```python
from build123d import *

# Parameters (mm, degrees)
BOSS_EXTRUDE1_DEPTH = 38.1
CUT_EXTRUDE1_DEPTH  = 7.62
CUT_EXTRUDE4_DEPTH  = 39.624


with BuildPart() as part:
    # Sketch2 → Boss-Extrude1 (new body)
    with BuildSketch(Plane(origin=(0, 0, 0), x_dir=(1, 0, 0), z_dir=(0, 1, 0))):
        with BuildLine():
            Line((-13.549240888, -8.64489), (-13.549240888, -32.77489))
            Line((-13.549240888, -32.77489), (21.502759112, -26.594276672))
            Line((21.502759112, -26.594276672), (21.502759112, -40.52189))
            Line((21.502759112, -40.52189), (478.702759112, -40.52189))
            ThreePointArc((478.702759112, -40.52189), (498.514759112, -20.70989), (478.702759112, -0.89789))
            Line((478.702759112, -0.89789), (21.502759112, -0.89789))
            Line((21.502759112, -0.89789), (21.502759112, -14.825503328))
            Line((21.502759112, -14.825503328), (-13.549240888, -8.64489))
        make_face()
    extrude(amount=BOSS_EXTRUDE1_DEPTH)

    # Sketch3 → Cut-Extrude1 (cut)
    with BuildSketch(Plane(origin=(0, 38.1, 0), x_dir=(1, 0, 0), z_dir=(0, 1, 0))):
        Polygon((-13.549240888, -8.64489), (-13.549240888, -32.77489), (21.502759112, -26.594276672), (21.502759112, -14.825503328), align=None)
    extrude(amount=-CUT_EXTRUDE1_DEPTH, mode=Mode.SUBTRACT)

    # Sketch5 → Cut-Extrude4 (cut)
    with BuildSketch(Plane.XY.offset(40.52189)):
        Polygon((250.102759112, 38.1), (498.514759112, 15.775221318), (498.514759112, 38.1), align=None)
    extrude(amount=-CUT_EXTRUDE4_DEPTH, mode=Mode.SUBTRACT)


solid = part.part
```
Geometry check sheet. Reference: the model listing, model coordinates, mm. A direction names the side the tool comes from. Coordinates: 2 decimals unless noted, no trailing zeros. Order: outer loops, then holes, each group sorted by start corner. A loop starts at its lowest first (then second) coordinate and runs counter-clockwise, first axis right, second up. Notation, with made-up numbers: (2, 49.25) - (38, 49.25) arc R33 cw to (38, 78.25) - close; hole circle Ø1 at (21.25, 73.5). An arc over 180 degrees is marked (long way). Answer in a Markdown table with one row per item. Add a question column.
1. Draft check along X on faces 4 (the face through (372.57, 27.094, 20.987)), 5 (the face through (4.22, 15.03, 11.78)), 6 (the face through (239, 0, 20)). Enter one of: +X half, -X half, draft (parallel to the pull), parting line (faces both ways), or undercut.
2. Section check A-A (y = 10). Enter the section's corners in (x, z), plus the area to 3 significant figures.
3. Section check B-B (x = 362). Enter the section's corners in (y, z), plus the area to 3 significant figures.
4. Section check C-C (x = 418). Enter the section's corners in (y, z).
5. Material ranges on L1, parallel to Y at x = 335.5, z = 5; L2, parallel to X at y = 5.5, z = 20; L3, parallel to Y at x = 423.5, z = 37, recorded low to high. Write a range as [from, to].
6. Gauge pin test, flat end, axial feed: pin 1 Ø12 at (x, z) = (422, 35.5) entering from +Y. Record the tip position at first contact, or that the pin passes through.
7. Access from +Z, -Z, +X, -X, +Y, -Y to the whole of each face (thin tool, end or side, straight path). Record for faces 1 (the face through (3.73, 15.03, 29.73)), 2 (the face through (498.51, 8.65, 21.15)), 3 (the face through (0, 30.48, 21)).
Data:
| question | item | result |
|---|---|---|
| 1 | face 4 | +X half |
| 1 | face 5 | undercut |
| 1 | face 6 | draft |
| 2 | outline | (-13.55, 8.64) - (21.5, 14.83) - (21.5, 0.9) - (478.7, 0.9) arc R19.81 ccw to (478.7, 40.52) - (21.5, 40.52) - (21.5, 26.59) - (-13.55, 32.77) - close |
| 2 | area | 19,400 mm² |
| 3 | outline | (0, 0.9) - (28.04, 0.9) - (28.04, 40.52) - (0, 40.52) - close |
| 3 | area | 1,110 mm² |
| 4 | outline | (0, 0.9) - (23.01, 0.9) - (23.01, 40.52) - (0, 40.52) - close |
| 5 | L1 | y = [0, 30.43] |
| 5 | L2 | x = [-13.55, 498.5] |
| 5 | L3 | y = [0, 22.52] |
| 6 | pin 1 | stops at y = 23.19 |
| 7 | face 1 | +Z, +Y, -Y |
| 7 | face 2 | +X, +Y, -Y |
| 7 | face 3 | +Z, -Z, -X, +Y |
